from build123d import *

# Parameters (mm, degrees)
SKETCH_1_R               = 1.2
EXTRUDE_1_DEPTH          = 10
SKETCH_3_W               = 10
SKETCH_3_H               = 15
EXTRUDE_2_DEPTH          = 2
FILLET_2_R               = 3
FILLET_START             = -5
FILLET_3_DEPTH           = 10
FILLET_START_2           = 2
FILLET_3_2_DEPTH         = 4.9438
FILLET_START_3           = -9
FILLET_3_3_DEPTH         = 17
SKETCH_4_W               = 15.92154
SKETCH_4_H               = 1.2
CUT_EXTRUDE_2_DEPTH      = 20.710403
CUT_EXTRUDE_4_DEPTH      = 19.227726
CUT_EXTRUDE_4_DEPTH_BACK = 1
SKETCH_6_R               = 1.95
SKETCH_7_R               = 1.15
CUT_EXTRUDE_5_DEPTH      = 19.794946
CUT_EXTRUDE_6_DEPTH      = 1


with BuildPart() as part:
    # 草图1 → 凸台-拉伸1 (new body)
    with BuildSketch(Plane(origin=(0, 0, 0), x_dir=(1, 0, 0), z_dir=(0, 1, 0))):
        with BuildLine():
            Line((-9, 2.5), (9, 2.5))
            ThreePointArc((9, 2.5), (11.5, 0), (9, -2.5))
            Line((9, -2.5), (-9, -2.5))
            ThreePointArc((-9, -2.5), (-11.5, 0), (-9, 2.5))
        make_face()
        with Locations(Location((9, 0, 0), (0, 0, 270))):
            Circle(SKETCH_1_R, mode=Mode.SUBTRACT)
        with Locations(Location((-9, 0, 0), (0, 0, 90))):
            Circle(SKETCH_1_R, mode=Mode.SUBTRACT)
    extrude(amount=EXTRUDE_1_DEPTH)

    # 草图3 → 凸台-拉伸2 (add)
    with BuildSketch(Plane.XZ):
        with Locations((0, 5)):
            Rectangle(SKETCH_3_W, SKETCH_3_H)
    extrude(amount=-EXTRUDE_2_DEPTH)

    # 圆角2
    fillet_2_edges = [part.edges().sort_by_distance(p)[0] for p in [
        (5, 1, 12.5),
        (5, 1, 2.5),
        (-5, 1, 2.5),
        (-5, 1, 12.5),
    ]]
    fillet(fillet_2_edges, radius=FILLET_2_R)

    # 圆角3: read off the stored shape, not the designer's step
    # 圆角3 outline → 圆角3 (add)
    with BuildSketch(Plane.YZ.offset(FILLET_START)):
        with BuildLine():
            ThreePointArc((7, 2.5), (3.464466, 3.964466), (2, 7.5))
            Line((2, 7.5), (2, 2.5))
            Line((2, 2.5), (7, 2.5))
        make_face()
    extrude(amount=FILLET_3_DEPTH)

    # Fillet 3 2 outline → Fillet 3 2 (add)
    with BuildSketch(Plane(origin=(0, 0, 0), x_dir=(1, 0, 0), z_dir=(0, 1, 0)).offset(FILLET_START_2)):
        with BuildLine():
            Line((5, -2.5), (5, -5.5))
            ThreePointArc((5, -5.5), (5.87868, -3.37868), (8, -2.5))
            Line((8, -2.5), (5, -2.5))
        make_face()
        with BuildLine():
            Line((-5, -5.5), (-5, -2.5))
            Line((-5, -2.5), (-8, -2.5))
            ThreePointArc((-8, -2.5), (-5.87868, -3.37868), (-5, -5.5))
        make_face()
    extrude(amount=FILLET_3_2_DEPTH)

    # Fillet 3 3 outline → Fillet 3 3 (cut)
    with BuildSketch(Plane.YZ.offset(FILLET_START_3)):
        with BuildLine():
            Line((8, 7), (2.025063, 7))
            ThreePointArc((2.025063, 7), (3.625111, 3.81081), (6.9438, 2.500316))
            ThreePointArc((6.9438, 2.500316), (6.9719, 2.500079), (7, 2.5))
            Line((7, 2.5), (8, 2.5))
            Line((8, 2.5), (8, 7))
        make_face()
    extrude(amount=FILLET_3_3_DEPTH, mode=Mode.SUBTRACT)

    # 草图4 → 切除-拉伸2 (cut, through all)
    with BuildSketch(Plane.XZ):
        Rectangle(SKETCH_4_W, SKETCH_4_H)
    extrude(amount=-CUT_EXTRUDE_2_DEPTH, mode=Mode.SUBTRACT)

    # 草图6 → 切除-拉伸4 (cut, two sides: drawn at the far end of the back side and taken through both)
    with BuildSketch(Plane.XY.offset(2.5).offset(-CUT_EXTRUDE_4_DEPTH_BACK)):
        with Locations(Location((0, 6, 0), (0, 0, 149.148114))):
            Circle(SKETCH_6_R)
    extrude(amount=CUT_EXTRUDE_4_DEPTH + CUT_EXTRUDE_4_DEPTH_BACK, mode=Mode.SUBTRACT)

    # 草图7 → 切除-拉伸5 (cut, through all)
    with BuildSketch(Plane.XY.offset(1.5)):
        with Locations((0, 6)):
            Circle(SKETCH_7_R)
    extrude(amount=-CUT_EXTRUDE_5_DEPTH, mode=Mode.SUBTRACT)

    # 草图8 → 切除-拉伸6 (cut)
    with BuildSketch(Plane(origin=(0, 0, -2.5), x_dir=(-1, 0, 0), z_dir=(0, 0, -1))):
        Polygon((0, 8.424871), (-2.1, 7.212436), (-2.1, 4.787564), (0, 3.575129), (2.1, 4.787564), (2.1, 7.212436), align=None)
    extrude(amount=-CUT_EXTRUDE_6_DEPTH, mode=Mode.SUBTRACT)


solid = part.part
For this review, take the finished solid that the model builds, in its own axes (mm). A direction names the side the tool comes from. Round coordinates to 2 decimals unless told otherwise and drop trailing zeros. Loops run counter-clockwise (first coordinate to the right, second up) from the corner with the lowest first, then second, coordinate; pieces in that order, holes last. Notation, with made-up numbers: (74.25, 57) - (86.25, 57) arc R6 cw to (86.25, 63) - close; hole circle Ø10 at (-31, 42.25). An arc over 180 degrees is marked (long way). Use one line per item in the form item = value.
1) Clearance check with flat-ended pins moving along their axes: P1, Ø1.8, axis at x = 0, y = 6, coming from the +Z side; P2, Ø3, axis at x = -7.5, y = 2, coming from the +Z side; P3, Ø2.5, axis at x = 0, z = 9.5, coming from the +Y side; P4, Ø3.5, axis at x = 0, y = 6, coming from the -Z side. State where each tip first meets the part, or that it passes through.
Solutions:
P1 = through
P2 = 3.26
P3 = 2
P4 = -1.5
2) Wall thickness on probe 1 along Z at (x, y) = (-5.25, 9.25); probe 2 along X at (y, z) = (1.25, 0.75); probe 3 along Y at (x, z) = (0, 1): over which ranges is each line inside the solid? List them lowest first.
Solutions:
probe_1 = -2.5 to -0.6, 0.6 to 2.5
probe_2 = -11.38 to -9.94, -8.06 to 8.06, 9.94 to 11.38
probe_3 = 0 to 4.85, 7.15 to 10
3) Tool access review of faces 4 (the face through (-1.065, 7.81, -2.007)), 5 (the face through (-11.5, 4.9, 0.1)): name each direction out of +Z, -Z, +X, -X, +Y, -Y from which nothing blocks a thin tool from reaching the whole face with its end or side.
Solutions:
face_4 = -Z
face_5 = -X, +Y, -Y
4) Mouldability with a two-part tool opening along Z and no side actions: class faces 1 (the face through (0, 4, 0.6)), 2 (the face through (-4.14, 1.01, 11.6)), 3 (the face through (-5, 1, 8)) as pulls with the +Z half, pulls with the -Z half, needs draft (parallel to the pull), parting line crosses it, or undercut.
Solutions:
face_1 = undercut
face_2 = pulls with the +Z half
face_3 = needs draft
5) We need section C-C on x = 3.25. Write out the cut boundary in (y, z), then the cut area to 3 significant figures.
Solutions:
outline = (0, -2.5) - (10, -2.5) - (10, -0.6) - (0, -0.6) - close; (0, 0.6) - (10, 0.6) - (10, 2.5) - (7, 2.5) arc R5 cw to (2, 7.5) - (2, 12.23) - (0, 12.23) - close
area = 62.8 mm2
6) We need section D-D on y = 6. Write out the cut boundary in (x, z).
Solutions:
outline = (-9, -2.5) - (-2.1, -2.5) - (-2.1, -1.5) - (-1.15, -1.5) - (-1.15, -0.6) - (-7.96, -0.6) arc R1.2 cw (long way) to (-7.96, 0.6) - (-1.15, 0.6) - (-1.15, 1.5) - (-1.95, 1.5) - (-1.95, 2.6) - (-7.23, 2.6) arc R3 cw to (-8, 2.5) - (-9, 2.5) arc R2.5 ccw to start; (1.15, -1.5) - (2.1, -1.5) - (2.1, -2.5) - (9, -2.5) arc R2.5 ccw to (9, 2.5) - (8, 2.5) arc R3 cw to (7.23, 2.6) - (1.95, 2.6) - (1.95, 1.5) - (1.15, 1.5) - (1.15, 0.6) - (7.96, 0.6) arc R1.2 cw (long way) to (7.96, -0.6) - (1.15, -0.6) - close
7) We need section B-B on z = 0. Write out the cut boundary in (x, y).
Solutions:
outline = (-11.5, 0) - (-10.2, 0) - (-10.2, 10) - (-11.5, 10) - close; (10.2, 0) - (11.5, 0) - (11.5, 10) - (10.2, 10) - close
8) We need section A-A on y = 1.75. Write out the cut boundary in (x, z).
Solutions:
outline = (-9, -2.5) - (9, -2.5) arc R2.5 ccw to (9, 2.5) - (8, 2.5) arc R3 cw to (5, 5.5) - (5, 9.5) arc R3 ccw to (2, 12.5) - (-2, 12.5) arc R3 ccw to (-5, 9.5) - (-5, 5.5) arc R3 cw to (-8, 2.5) - (-9, 2.5) arc R2.5 ccw to start; hole (-7.96, -0.6) - (7.96, -0.6) arc R1.2 ccw (long way) to (7.96, 0.6) - (-7.96, 0.6) arc R1.2 ccw (long way) to start
